Verification items for the finished model (mm, model axes). A direction names the side the tool comes from. Give positions to 0.01 mm unless a question says otherwise; leave off trailing zeros. Order: outer loops, then holes, each group sorted by start corner. A loop starts at its lowest first (then second) coordinate and runs counter-clockwise, first axis right, second up. Notation, with made-up numbers: (-25, -10.5) - (33, -10.5) arc R27 ccw to (33, 19.5) - close; hole circle Ø3 at (76, 34). An arc over 180 degrees is marked (long way). Answer as a JSON object with one key per item and string values. Group by question number.
(1) Mould release check, pull along Z, two halves, no side actions. Record for faces 1 (the face through (-25, 3, 61)), 2 (the face through (-1, 0, -1)), 3 (the face through (-3.4, 6.5, -86.2)), 4 (the face through (0, 2, -95)): +Z half, -Z half, draft (parallel to the pull), parting line (faces both ways), or undercut.
(2) Access from +Z, -Z, +X, -X, +Y, -Y to the whole of each face (thin tool, end or side, straight path). Record for faces 5 (the face through (-22.44, 11, -84)), 6 (the face through (-0.32, 6.53, -86.42)), 7 (the face through (5, 8.1, -86)).
(3) Section check A-A (z = 77.5). Record the boundary of the cut face in (x, y), then the cut area to 3 significant figures.
(4) Section check B-B (y = 11). Record the boundary of the cut face in (x, z), then the cut area to 3 significant figures.
(5) Section check C-C (z = 6). Record the boundary of the cut face in (x, y), then the cut area to 3 significant figures.
(6) Thickness scan on line 1 (X direction, y = 4.25, z = 47); line 2 (X direction, y = 0.75, z = 72); line 3 (Z direction, x = 1.5, y = 14.5). Record the ranges inside material, lowest first.
(7) Section check D-D (x = 48). Record the boundary of the cut face in (y, z), then the cut area to 3 significant figures.
(8) Depth check by flat-ended pin: pin 1 Ø8 at (x, z) = (-3, -87.5) entering from +Y; pin 2 Ø2.5 at (y, z) = (11, -86) entering from +X; pin 3 Ø1 at (x, z) = (-19.5, -58.5) entering from +Y; pin 4 Ø1 at (y, z) = (6, -37) entering from -X. Enter the tip coordinate at first touch or a pass-through.
```python
from build123d import *

# Parameters (mm, degrees)
SKETCH1_W                = 90
SKETCH1_H                = 190
BOSS_EXTRUDE1_DEPTH      = 5
SKETCH2_W                = 10
SKETCH2_H                = 30
BOSS_EXTRUDE2_DEPTH      = 5
CHAMFER1_SIZE            = 2
SKETCH3_W                = 16
SKETCH3_H                = 34
CUT_EXTRUDE1_DEPTH       = 50
SKETCH4_W                = 90
SKETCH4_H                = 42
CUT_EXTRUDE2_DEPTH       = 1
SKETCH7_W                = 15.1
SKETCH7_H                = 89.916335477
CUT_EXTRUDE7_DEPTH       = 1
CUT_EXTRUDE9_DEPTH       = 110.886304879
CUT_EXTRUDE9_DEPTH_BACK  = 110.886304879
CUT_EXTRUDE10_DEPTH      = 110.886304879
CUT_EXTRUDE10_DEPTH_BACK = 110.886304879
BOSS_EXTRUDE4_START      = 5
SKETCH17_W               = 2.5
SKETCH17_H               = 8
BOSS_EXTRUDE4_DEPTH      = 13
BOSS_EXTRUDE5_DEPTH      = 3.1
CUT_EXTRUDE11_START      = 5
CUT_EXTRUDE11_DEPTH      = 1


with BuildPart() as part:
    # Sketch1 → Boss-Extrude1 (new body)
    with BuildSketch(Plane(origin=(0, 0, 0), x_dir=(1, 0, 0), z_dir=(0, 1, 0))):
        Rectangle(SKETCH1_W, SKETCH1_H)
    extrude(amount=BOSS_EXTRUDE1_DEPTH)

    # Sketch2 → Boss-Extrude2 (add)
    with BuildSketch(Plane(origin=(0, 0, 0), x_dir=(1, 0, 0), z_dir=(0, 1, 0))):
        with Locations((-50, -80)):
            Rectangle(SKETCH2_W, SKETCH2_H)
        with Locations((50, -80)):
            Rectangle(SKETCH2_W, SKETCH2_H)
    extrude(amount=BOSS_EXTRUDE2_DEPTH)

    # Chamfer1
    chamfer1_edges = [part.edges().sort_by_distance(p)[0] for p in [
        (-55, 2.5, 65),
        (-55, 2.5, 95),
        (55, 2.5, 95),
        (55, 2.5, 65),
    ]]
    chamfer(chamfer1_edges, length=CHAMFER1_SIZE)

    # Sketch3 → Cut-Extrude1 (cut)
    with BuildSketch(Plane(origin=(0, 5, 0), x_dir=(1, 0, 0), z_dir=(0, 1, 0))):
        with Locations((-25, -78)):
            Rectangle(SKETCH3_W, SKETCH3_H)
    extrude(amount=-CUT_EXTRUDE1_DEPTH, mode=Mode.SUBTRACT)

    # Sketch4 → Cut-Extrude2 (cut)
    with BuildSketch(Plane(origin=(0, 5, 0), x_dir=(1, 0, 0), z_dir=(0, 1, 0))):
        with Locations((0, 59.159820088)):
            Rectangle(SKETCH4_W, SKETCH4_H)
    extrude(amount=-CUT_EXTRUDE2_DEPTH, mode=Mode.SUBTRACT)

    # Sketch7 → Cut-Extrude7 (cut)
    with BuildSketch(Plane(origin=(0, 5, 0), x_dir=(1, 0, 0), z_dir=(0, 1, 0))):
        with Locations((37.45, -15.495273531)):
            Rectangle(SKETCH7_W, SKETCH7_H)
        with Locations((0.16773297, -15.495273531)):
            Rectangle(SKETCH7_W, SKETCH7_H)
    extrude(amount=-CUT_EXTRUDE7_DEPTH, mode=Mode.SUBTRACT)

    # Sketch14 → Cut-Extrude9 (cut, two sides: drawn at the far end of the back side and taken through both)
    with BuildSketch(Plane(origin=(0, 0, 0), x_dir=(1, 0, 0), z_dir=(0, 1, 0)).offset(-CUT_EXTRUDE9_DEPTH_BACK)):
        with BuildLine():
            Line((-45, 47.267125731), (-34.685032462, 30.799006468))
            ThreePointArc((-34.685032462, 30.799006468), (-34.351546651, 18.443044928), (-45, 12.166784925))
            Line((-45, 12.166784925), (-45, 47.267125731))
        make_face()
        with BuildLine():
            Line((45, 47.267125731), (45, 12.166784925))
            ThreePointArc((45, 12.166784925), (34.351546651, 18.443044928), (34.685032462, 30.799006468))
            Line((34.685032462, 30.799006468), (45, 47.267125731))
        make_face()
    extrude(amount=CUT_EXTRUDE9_DEPTH + CUT_EXTRUDE9_DEPTH_BACK, mode=Mode.SUBTRACT)

    # Sketch16 → Cut-Extrude10 (cut, two sides: drawn at the far end of the back side and taken through both)
    with BuildSketch(Plane(origin=(0, 0, 0), x_dir=(1, 0, 0), z_dir=(0, 1, 0)).offset(-CUT_EXTRUDE10_DEPTH_BACK)):
        with BuildLine():
            Line((-32.828659242, 95), (-32.828659242, 24.338125683))
            ThreePointArc((-32.828659242, 24.338125683), (-33.30195485, 27.699267678), (-34.685032462, 30.799006468))
            Line((-34.685032462, 30.799006468), (-45, 47.267125731))
            Line((-45, 47.267125731), (-45, 95))
            Line((-45, 95), (-32.828659242, 95))
        make_face()
        with BuildLine():
            Line((45, 95), (32.828659242, 95))
            Line((32.828659242, 95), (32.828659242, 24.338125683))
            ThreePointArc((32.828659242, 24.338125683), (33.30195485, 27.699267678), (34.685032462, 30.799006468))
            Line((34.685032462, 30.799006468), (45, 47.267125731))
            Line((45, 47.267125731), (45, 95))
        make_face()
    extrude(amount=CUT_EXTRUDE10_DEPTH + CUT_EXTRUDE10_DEPTH_BACK, mode=Mode.SUBTRACT)

    # Sketch17 → Boss-Extrude4 (add)
    with BuildSketch(Plane(origin=(0, 0, 0), x_dir=(1, 0, 0), z_dir=(0, 1, 0)).offset(BOSS_EXTRUDE4_START)):
        with Locations((-21.190023983, 84.159820088)):
            Rectangle(SKETCH17_W, SKETCH17_H)
        Polygon((-22.440023983, 94.999820088), (-22.440023983, 92.499820088), (18.940023983, 92.499820088), (19.940023983, 91.499820088), (19.940023983, 80.159820088), (22.440023983, 80.159820088), (22.440023983, 92.535353994), (19.975557889, 94.999820088), align=None)
    extrude(amount=BOSS_EXTRUDE4_DEPTH)

    # Sketch18 → Boss-Extrude5 (add)
    with BuildSketch(Plane(origin=(0, 5, 0), x_dir=(1, 0, 0), z_dir=(0, 1, 0))):
        Polygon((-12.599634528, 80.159820088), (-10.599634528, 80.159820088), (-6.108241837, 92.499820088), (-8.108241837, 92.499820088), align=None)
        Polygon((-3.108241837, 92.499820088), (-7.599634528, 80.159820088), (-5.599634528, 80.159820088), (-1.108241837, 92.499820088), align=None)
        Polygon((1.891758163, 92.499820088), (-2.599634528, 80.159820088), (-0.599634528, 80.159820088), (3.891758163, 92.499820088), align=None)
        Polygon((6.891758163, 92.499820088), (2.400365472, 80.159820088), (4.400365472, 80.159820088), (8.891758163, 92.499820088), align=None)
        Polygon((11.891758163, 92.499820088), (7.400365472, 80.159820088), (9.400365472, 80.159820088), (13.891758163, 92.499820088), align=None)
    extrude(amount=BOSS_EXTRUDE5_DEPTH)

    # Sketch19 → Cut-Extrude11 (cut)
    with BuildSketch(Plane(origin=(0, 0, 0), x_dir=(1, 0, 0), z_dir=(0, 1, 0)).offset(CUT_EXTRUDE11_START)):
        Polygon((-35, -65), (-35, -70), (-40.5, -70), (-40.5, -90), (-35, -90), (-35, -95), (-53, -95), (-55, -93), (-55, -67), (-53, -65), align=None)
    cut_extrude11 = extrude(amount=-CUT_EXTRUDE11_DEPTH, mode=Mode.SUBTRACT)

    # Mirror1: Cut-Extrude11 across plane
    add(cut_extrude11.mirror(Plane(origin=(0, 0, 0), x_dir=(0, 0, 1), z_dir=(1, 0, 0))), mode=Mode.SUBTRACT)


solid = part.part
```
Solutions:
{
 "1": {"face 1": "+Z half", "face 2": "draft", "face 3": "undercut", "face 4": "-Z half"},
 "2": {"face 5": "+Z, -Z, -X, +Y", "face 6": "+Y", "face 7": "+Z, +Y"},
 "3": {"outline": "(-55, 0) - (-33, 0) - (-33, 5) - (-40.5, 5) - (-40.5, 4) - (-55, 4) - close; (-17, 0) - (55, 0) - (55, 4) - (40.5, 4) - (40.5, 5) - (-17, 5) - close", "area": "441 mm2"},
 "4": {"outline": "(-22.44, -95) - (19.98, -95) - (22.44, -92.54) - (22.44, -80.16) - (19.94, -80.16) - (19.94, -91.5) - (18.94, -92.5) - (-22.44, -92.5) - close; (-22.44, -88.16) - (-19.94, -88.16) - (-19.94, -80.16) - (-22.44, -80.16) - close", "area": "161 mm2"},
 "5": {"outline": "(-45, 0) - (45, 0) - (45, 4) - (29.9, 4) - (29.9, 5) - (7.72, 5) - (7.72, 4) - (-7.38, 4) - (-7.38, 5) - (-45, 5) - close", "area": "420 mm2"},
 "6": {"line 1": "x = -45 to -7.38, 7.72 to 29.9", "line 2": "x = -55 to -33, -17 to 55", "line 3": "z = -95 to -92.5"},
 "7": {"outline": "(0, 65) - (4, 65) - (4, 95) - (0, 95) - close", "area": "120 mm2"},
 "8": {"pin 1": "stops at y = 8.1", "pin 2": "stops at x = 22.44", "pin 3": "stops at y = 4", "pin 4": "passes through"}
}
